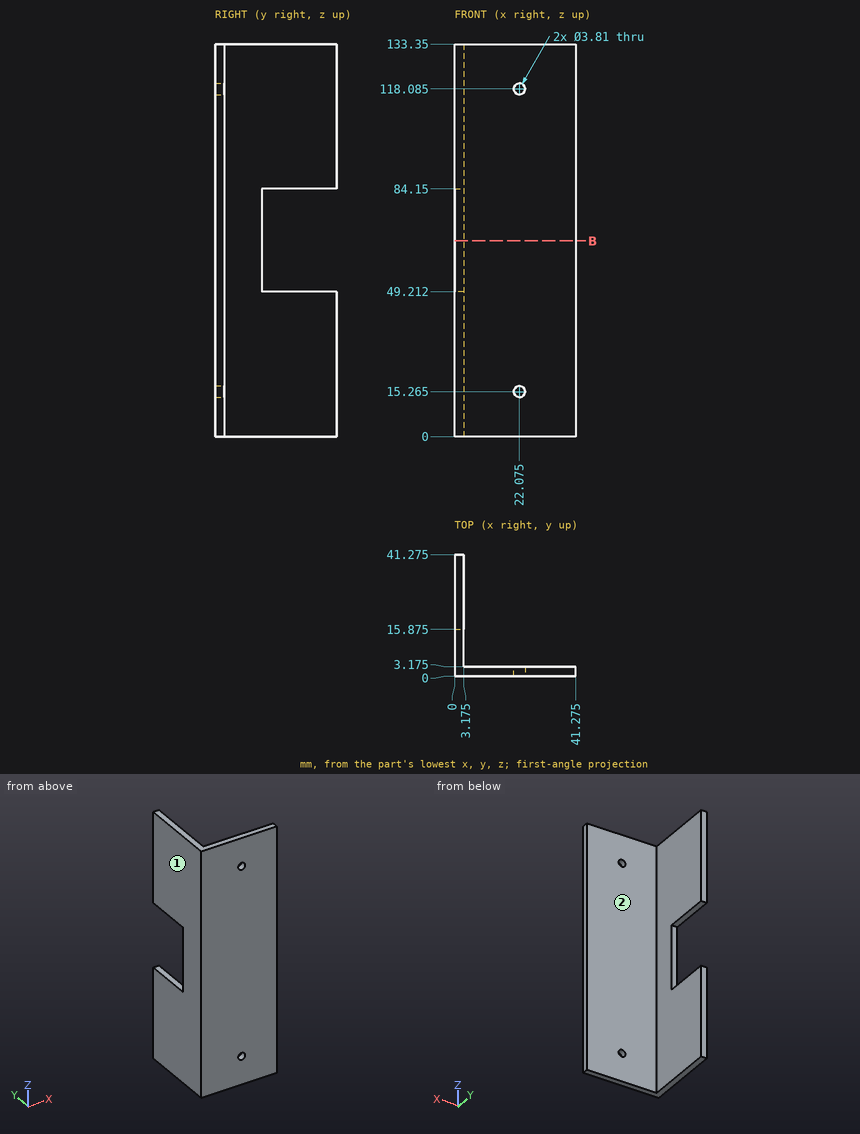
Design review of the part shown in the three views and the two pictorial views. Dimensions are in mm from the part's minimum x, y and z. A direction names the side the tool comes from. Coordinates: 2 decimals unless noted, no trailing zeros. Loops run counter-clockwise (first coordinate to the right, second up) from the corner with the lowest first, then second, coordinate; pieces in that order, holes last.
Q1. For pin 1 (2.5 mm diameter, centred on x = 2, y = 29.5, fed in from -Z); pin 2 (19 mm diameter, centred on y = 24.5, z = 43, fed in from +X) (1 decimal); pin 3 (2.5 mm diameter, centred on x = 2, z = 67, fed in from +Y) (1 decimal); pin 4 (10 mm diameter, centred on x = 19, z = 93.5, fed in from +Y) (1 decimal), all flat-tipped, find the tip position at first contact; note any pin that passes through.
Reported:
pin 1: stops at z = 0
pin 2: stops at x = 3.2
pin 3: stops at y = 15.9
pin 4: stops at y = 3.2
Q2. Tool access review of the marked faces 1 and 2: name each direction out of +Z, -Z, +X, -X, +Y, -Y from which nothing blocks a thin tool from reaching the whole face with its end or side.
Reported:
face 1: +Z, -Z, -X, +Y, -Y
face 2: +Z, -Z, +X, +Y
Q3. We need section B-B on z = 66.5. State the section outline as (x, y) points (1 decimal), and give its area (3 significant figures).
Reported:
outline: (0, 0) - (41.3, 0) - (41.3, 3.2) - (3.2, 3.2) - (3.2, 15.9) - (0, 15.9) - close
area: 171 mm2
Q4. To check wall thickness, follow line 1 (Z direction, x = 2, y = 28.5); line 2 (Y direction, x = 3.5, z = 45) (1 decimal). State the ranges of each line that lie inside material, in increasing order.
Reported:
line 1: z = 0 to 49.21, 84.15 to 133.35
line 2: y = 0 to 3.2
